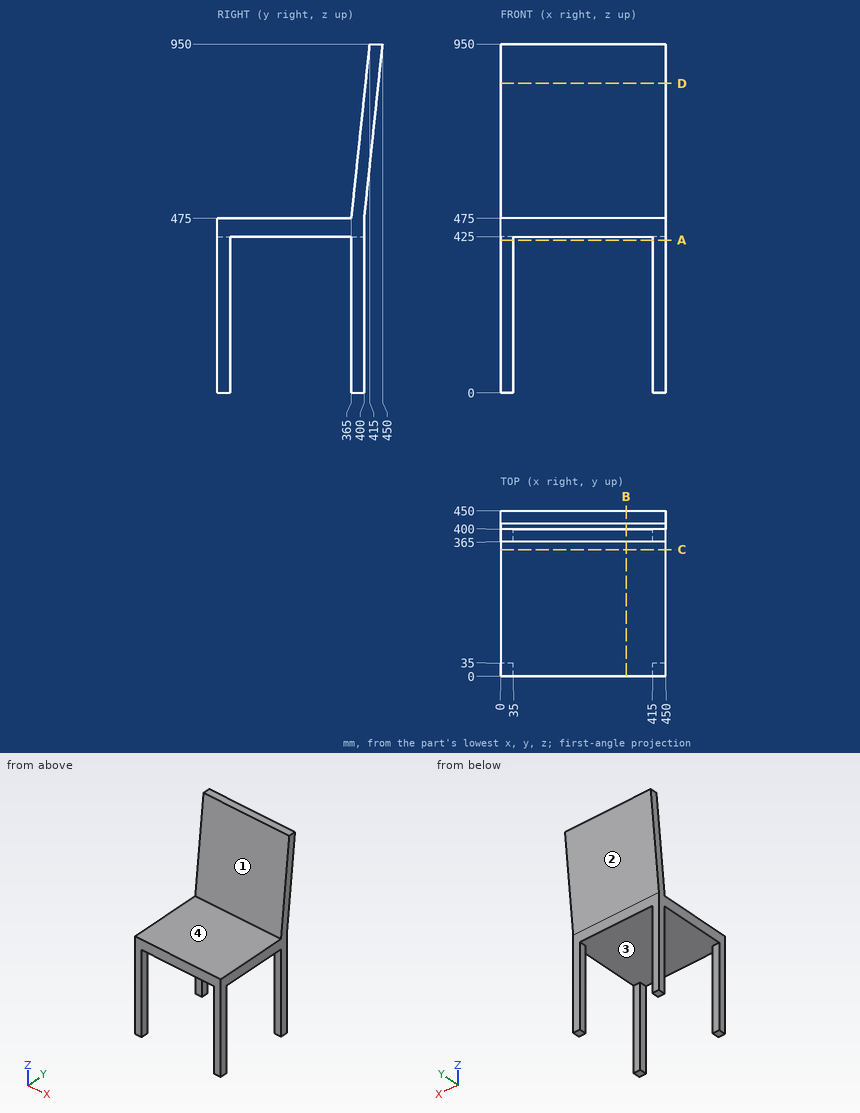
Drawing for the job (mm, zero at the part's lowest x, y, z). Round coordinates to 2 decimals unless told otherwise and drop trailing zeros. Loops run counter-clockwise (first coordinate to the right, second up) from the corner with the lowest first, then second, coordinate; pieces in that order, holes last. Notation, with made-up numbers: (16.5, 6) - (65.5, 6) arc R20 cw to (65.5, 17) - close; hole circle Ø8 at (5, 76.25). An arc over 180 degrees is marked (long way). Return JSON: item names as keys, results as strings. Group by question number.
Q1. Drill centre lines: line 1 along Z through (x, y) = (214, 25); line 2 along Y through (x, z) = (214.5, 505); line 3 along Y through (x, z) = (273.5, 854). Where is each one in solid material? Low to high. Write a range as [from, to].
Q2. Band-saw the part on A-A on z = 415.5. Give the cut face in (x, y).
Q3. Band-saw the part on D-D on z = 842.5. Give the cut face in (x, y).
Q4. Two-plate mould, pull along Y, no slides. Class the marked faces 1, 2, 3 and 4: +Y half, -Y half, draft (parallel to the pull), parting line (faces both ways), or undercut.
Q5. Band-saw the part on C-C on y = 344. Give the cut face in (x, z).
Q6. Flat gauge pins, fed straight in: pin 1 Ø5 at (x, z) = (315, 566.5) entering from +Y; pin 2 Ø17.5 at (x, z) = (430, 214) entering from +Y; pin 3 Ø1.5 at (x, z) = (282.5, 608.5) entering from -Y; pin 4 Ø10.5 at (x, z) = (439.5, 271) entering from -Y. Where does each tip first touch, or does it go through?
Q7. Band-saw the part on B-B on x = 342. Give the cut face in (y, z), plus the area to 3 significant figures.
Solutions:
{
 "1": {"line 1": "z = [425, 475]", "line 2": "y = [368.16, 403.16]", "line 3": "y = [404.89, 439.89]"},
 "2": {"outline": "(0, 0) - (35, 0) - (35, 35) - (0, 35) - close; (0, 365) - (35, 365) - (35, 400) - (0, 400) - close; (415, 0) - (450, 0) - (450, 35) - (415, 35) - close; (415, 365) - (450, 365) - (450, 400) - (415, 400) - close"},
 "3": {"outline": "(0, 403.68) - (450, 403.68) - (450, 438.68) - (0, 438.68) - close"},
 "4": {"face 1": "-Y half", "face 2": "+Y half", "face 3": "undercut", "face 4": "draft"},
 "5": {"outline": "(0, 425) - (450, 425) - (450, 475) - (0, 475) - close"},
 "6": {"pin 1": "stops at y = 409.89", "pin 2": "stops at y = 400", "pin 3": "stops at y = 378.97", "pin 4": "stops at y = 0"},
 "7": {"outline": "(0, 425) - (400, 425) - (400, 475) - (450, 950) - (415, 950) - (365, 475) - (0, 475) - close", "area": "36,600 mm^2"}
}
